from build123d import *

# Parameters (mm, degrees)
F0_R     = 22.5
F1_DEPTH = 25
F2_R     = 19.5
F3_DEPTH = 25.001
F5_DEPTH = 25


with BuildPart() as f1:
    # F0 (on Top) → F1 (new body)
    with BuildSketch(Plane.XY):
        Circle(F0_R)
    extrude(amount=F1_DEPTH)

    # F2 (on Top) → F3 (cut, through all)
    with BuildSketch(Plane.XY):
        Circle(F2_R)
    extrude(amount=F3_DEPTH, mode=Mode.SUBTRACT)

    # F4 (on face) → F5 (join)
    with BuildSketch(Plane(origin=(0, 0, 0), x_dir=(1, 0, 0), z_dir=(0, 0, -1))):
        with BuildLine():
            Line((-30, -22.5), (5.03e-08, -22.5))
            ThreePointArc((5.03e-08, -22.5), (-22.5, -1.28e-08), (2.47e-08, 22.5))
            Line((2.47e-08, 22.5), (-30, 22.5))
            Line((-30, 22.5), (-30, -22.5))
        make_face()
        with BuildLine():
            Line((5.03e-08, -22.5), (30, -22.5))
            Line((30, -22.5), (30, 22.5))
            Line((30, 22.5), (2.47e-08, 22.5))
            ThreePointArc((2.47e-08, 22.5), (15.9099025854, 15.909902568), (22.5, 0))
            ThreePointArc((22.5, 0), (15.9099025945, -15.9099025589), (5.03e-08, -22.5))
        make_face()
    extrude(amount=-F5_DEPTH)


solid = f1.part
CAD build for the part. Positions are in the model's coordinates, mm. Give positions to 0.01 mm unless a question says otherwise; leave off trailing zeros. Write each loop counter-clockwise with the first axis right and the second up, starting at its lowest first coordinate (ties: lowest second). Pieces come first, ordered by that corner, then holes. Notation, with made-up numbers: M 33.5,48.25 L 51.5,48.25 A7 cw 51.5,58.25 Z; hole C 65,-19 d4. An arc over 180 degrees is marked long. Put each result on its own line as item: value. Start each with the question number.
(1) Probe L1, parallel to Y at x = 0, z = 10; L2, parallel to X at y = 0, z = 6.75; L3, parallel to X at y = -3.5, z = 23. List the from-to ranges inside material, lowest first.
(2) Mould opens along X. For faces 1 (the face through (30, 0, 12)), 2 (the face through (-2.539, 19.334, 12.325)), 3 (the face through (-20, 0, 25)) say: +X half, -X half, draft (parallel to the pull), parting line (faces both ways), or undercut.
(3) Band-saw the part on B-B, the plane x = 0. Write the cut outline in (y, z).
(4) Band-saw the part on A-A, the plane y = 0. Write the cut outline in (x, z), and give its area (3 significant figures).
(5) Band-saw the part on C-C, the plane z = 22.5. Write the cut outline in (x, y), and give its area (3 significant figures).
Response values:
1. L1: y = -22.5 to -19.5, 19.5 to 22.5
1. L2: x = -30 to -19.5, 19.5 to 30
1. L3: x = -30 to -19.18, 19.18 to 30
2. face 1: +X half
2. face 2: undercut
2. face 3: draft
3. outline: M -22.5,0 L -19.5,0 L -19.5,25 L -22.5,25 Z; M 19.5,0 L 22.5,0 L 22.5,25 L 19.5,25 Z
4. outline: M -30,0 L -19.5,0 L -19.5,25 L -30,25 Z; M 19.5,0 L 30,0 L 30,25 L 19.5,25 Z
4. area: 525 mm2
5. outline: M -30,-22.5 L 30,-22.5 L 30,22.5 L -30,22.5 Z; hole C 0,0 d39
5. area: 1,510 mm2
